```python
from build123d import *

# Parameters (mm, degrees)
SKETCH2_W               = 22.86
SKETCH2_H               = 3.2258
CUT_EXTRUDE1_DEPTH      = 2.6035
CUT_EXTRUDE2_DEPTH      = 2.6035
SKETCH4_R               = 9.525
CUT_EXTRUDE3_DEPTH      = 16.494
CUT_EXTRUDE3_DEPTH_BACK = 16.494


with BuildPart() as part:
    # Sketch1 → Revolve1 (revolve)
    with BuildSketch(Plane.XY):
        with BuildLine():
            Line((0, 15.494), (0, -15.494))
            ThreePointArc((0, -15.494), (-15.494, 0), (0, 15.494))
        make_face()
    revolve(axis=Axis((0, 15.494, 0), (0, -1, 0)))

    # Sketch2 → Cut-Extrude1 (cut, symmetric)
    with BuildSketch(Plane.XY):
        with Locations((0, 13.8811)):
            Rectangle(SKETCH2_W, SKETCH2_H)
    extrude(amount=CUT_EXTRUDE1_DEPTH, both=True, mode=Mode.SUBTRACT)

    # Sketch3 → Cut-Extrude2 (cut, symmetric)
    with BuildSketch(Plane.XY):
        with BuildLine():
            Line((-9.463366, 12.2682), (9.463366, 12.2682))
            ThreePointArc((9.463366, 12.2682), (0, 9.930055), (-9.463366, 12.2682))
        make_face()
    extrude(amount=CUT_EXTRUDE2_DEPTH, both=True, mode=Mode.SUBTRACT)

    # Sketch4 → Cut-Extrude3 (cut, two sides)
    with BuildSketch(Plane.XY) as cut_extrude3_sk:
        Circle(SKETCH4_R)
    extrude(amount=CUT_EXTRUDE3_DEPTH, mode=Mode.SUBTRACT)
    extrude(cut_extrude3_sk.sketch, amount=-CUT_EXTRUDE3_DEPTH_BACK, mode=Mode.SUBTRACT)


solid = part.part
```
Verification items for the finished model (mm, model axes). Round coordinates to 2 decimals unless told otherwise and drop trailing zeros. Write each loop counter-clockwise with the first axis right and the second up, starting at its lowest first coordinate (ties: lowest second). Pieces come first, ordered by that corner, then holes. Notation, with made-up numbers: (-8.75, -30.5) -> (20.25, -30.5) arc R27 cw to (20.25, -14.5) -> close; hole circle Ø9 at (-22.5, 56). An arc over 180 degrees is marked (long way). Write each question's results on one line, items separated by ' | '. Start each with the question number.
1. Material ranges on probe 1 along Y at (x, z) = (4, -9.25); probe 2 along Y at (x, z) = (-7, -10); probe 3 along X at (y, z) = (0, 6) (3 decimals), recorded low to high. Write a range as from..to.
2. Cross-section at A-A (x = 0). Enter the section's corners in (y, z) (1 decimal).
3. Cross-section at C-C (z = -7.25). Enter the section's corners in (x, y) (3 decimals).
4. Depth check by flat-ended pin: P1, Ø4.5, axis at x = 3, y = 13.5, coming from the -Z side; P2, Ø1, axis at x = -9, y = -7.5, coming from the -Z side; P3, Ø1.5, axis at y = -7, z = 7, coming from the -X side. Enter the tip coordinate at first touch or a pass-through.
5. Cross-section at B-B (y = 0). Enter the section's corners in (x, z) (3 decimals), then the cut area to 3 significant figures.
6. Cross-section at D-D (x = 5). Enter the section's corners in (y, z).
7. Draft check along X on faces 1 (the cylindrical face through (-7.559, -5.796, 0.171)), 2 (the flat face through (0, 13, 2.604)). Enter one of: +X half, -X half, draft (parallel to the pull), parting line (faces both ways), or undercut.
Solutions:
1) probe 1: y = -11.77..-8.64, 8.64..11.77 | probe 2: y = -9.54..-6.46, 6.46..9.54 | probe 3: x = -14.285..-9.525, 9.525..14.285
2) outline: (-9.5, -12.2) -> (-9.5, 12.2) arc R15.5 ccw to start; (9.5, -12.2) arc R15.5 ccw to (15.3, -2.6) -> (9.9, -2.6) -> (9.9, 2.6) -> (15.3, 2.6) arc R15.5 ccw to (9.5, 12.2) -> close
3) outline: circle Ø27.386 at (0, 0); hole circle Ø19.05 at (0, 0)
4) P1: stops at z = -10.29 | P2: stops at z = -10.69 | P3: stops at x = -12.5
5) outline: (-9.525, -12.22) -> (-9.525, 12.22) arc R15.494 ccw to start; (9.525, -12.22) arc R15.494 ccw to (9.525, 12.22) -> close | area: 204 mm2
6) outline: (-8.11, -12.22) -> (-8.11, 12.22) arc R14.67 ccw to start; (8.11, -12.22) arc R14.67 ccw to (14.43, -2.6) -> (10.55, -2.6) -> (10.55, 2.6) -> (14.43, 2.6) arc R14.67 ccw to (8.11, 12.22) -> close
7) face 1: undercut | face 2: undercut
